Verification items for the finished model (mm, model axes). Coordinates: 2 decimals unless noted, no trailing zeros. Order: outer loops, then holes, each group sorted by start corner. A loop starts at its lowest first (then second) coordinate and runs counter-clockwise, first axis right, second up. Notation, with made-up numbers: (77.25, -19) - (92.25, -19) arc R31 ccw to (92.25, 13) - close; hole circle Ø3 at (-37.75, 42). An arc over 180 degrees is marked (long way). Answer as CSV lines item,"result". Start each with the question number.
1. Material ranges on L1, parallel to Z at x = 0, y = -4 (3 decimals); L2, parallel to X at y = -2.5, z = 146.05 (3 decimals); L3, parallel to X at y = -0.25, z = 151.5, recorded low to high. Write a range as [from, to].
2. Section check A-A (x = 0). Record the cut outline in (y, z) (3 decimals).
3. Section check B-B (y = -4). Record the cut outline in (x, z) (3 decimals), and give its area (3 significant figures).
4. Section check C-C (z = -146.05). Record the cut outline in (x, y) (3 decimals), and give its area (3 significant figures).
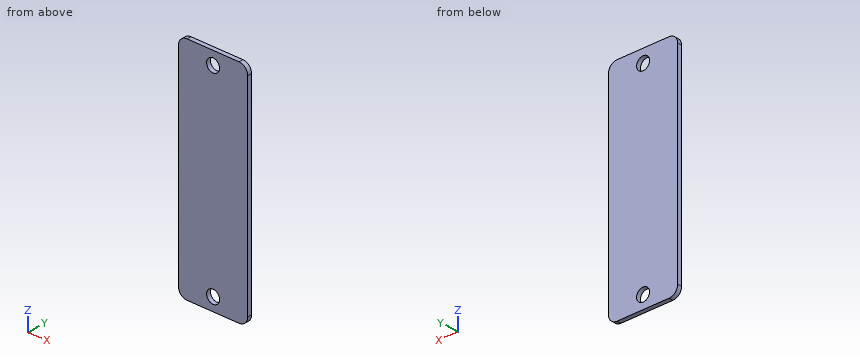
from build123d import *

# Parameters (mm, degrees)
F0_W     = 101.6
F0_H     = 330.2
F1_DEPTH = 6.35
F2_R     = 12.7
F4_D     = 19.05


with BuildPart() as f1:
    # F0 (on Front) → F1 (new body)
    with BuildSketch(Plane.XZ):
        Rectangle(F0_W, F0_H)
    extrude(amount=F1_DEPTH)

    # F2
    f2_edges = [f1.edges().sort_by_distance(p)[0] for p in [
        (50.8, -3.175, 165.1),
        (-50.8, -3.175, 165.1),
        (50.8, -3.175, -165.1),
        (-50.8, -3.175, -165.1),
    ]]
    fillet(f2_edges, radius=F2_R)

    # F4 (through all)
    with Locations(Plane(origin=(0, 0, 0), x_dir=(1, 0, 0), z_dir=(0, 1, 0))):
        with Locations((0, 146.05), (0, -146.05)):
            Hole(F4_D / 2)


solid = f1.part
Evaluation:
1,L1,"z = [-165.1, -155.575], [-136.525, 136.525], [155.575, 165.1]"
1,L2,"x = [-50.8, -9.525], [9.525, 50.8]"
1,L3,"x = [-50.8, -7.81], [7.81, 50.8]"
2,outline,"(-6.35, -165.1) - (0, -165.1) - (0, -155.575) - (-6.35, -155.575) - close; (-6.35, -136.525) - (0, -136.525) - (0, 136.525) - (-6.35, 136.525) - close; (-6.35, 155.575) - (0, 155.575) - (0, 165.1) - (-6.35, 165.1) - close"
3,outline,"(-50.8, -152.4) arc R12.7 ccw to (-38.1, -165.1) - (38.1, -165.1) arc R12.7 ccw to (50.8, -152.4) - (50.8, 152.4) arc R12.7 ccw to (38.1, 165.1) - (-38.1, 165.1) arc R12.7 ccw to (-50.8, 152.4) - close; hole circle Ø19.05 at (0, -146.05); hole circle Ø19.05 at (0, 146.05)"
3,area,"32,800 mm²"
4,outline,"(-50.8, -6.35) - (-9.525, -6.35) - (-9.525, 0) - (-50.8, 0) - close; (9.525, -6.35) - (50.8, -6.35) - (50.8, 0) - (9.525, 0) - close"
4,area,"524 mm²"
